Work out the finished part from the listing and answer in its coordinate system (mm). Round coordinates to 2 decimals unless told otherwise and drop trailing zeros. Loops run counter-clockwise (first coordinate to the right, second up) from the corner with the lowest first, then second, coordinate; pieces in that order, holes last. Notation, with made-up numbers: (32, -11.75) -> (50, -11.75) arc R21 ccw to (50, 0.25) -> close; hole circle Ø4 at (-19, 46). An arc over 180 degrees is marked (long way). Use one line per item in the form item = value.
Autodesk Inventor part; units mm, degrees
ref_plane "YZ Plane" through (0, 0, 0) normal (1, 0, 0) x (0, 1, 0)
ref_plane "XZ Plane" through (0, 0, 0) normal (0, 1, 0) x (-1, 0, 0)
ref_plane "XY Plane" through (0, 0, 0) normal (0, 0, 1) x (1, 0, 0)
sketch "Sketch1" plane through (0, 0, 0) normal (0, 1, 0) x (-1, 0, 0)
  line L0 (0, 0) -> (558.8, 0)
  line L1 (558.8, 0) -> (558.8, 79.375)
  line L2 (558.8, 79.375) -> (0, 79.375)
  line L3 (0, 79.375) -> (0, 0)
  dimension "d0" = 79.375
  dimension "d1" = 558.8
extrude "Extrusion1" add sketch "Sketch1" along normal blind 3.175
sketch "Sketch3" plane through (-558.8, 0, 0) normal (-1, 0, 0) x (0, 0, 1)
  line L0 (0, 0) -> (79.375, 0)
  line L1 (79.375, 0) -> (79.375, 3.175)
  line L2 (0, 3.175) -> (79.375, 3.175)
  line L3 (0, 0) -> (0, 3.175)
  line L4 (73.025, 3.175) -> (73.025, 0)
  line L5 (60.325, 0) -> (60.325, 3.175)
  line L6 (19.05, 0) -> (19.05, 3.175)
  line L7 (6.35, 0) -> (6.35, 3.175)
  dimension "d4" = 12.7
  dimension "d5" = 6.35
  dimension "d6" = 12.7
  dimension "d7" = 6.35
extrude "Extrusion2" cut sketch "Sketch3" against normal blind 3.175 contours L7 L2 L6 L0 | L5 L2 L4 L0
sketch "Sketch4" plane through (0, 0, 79.375) normal (1, 0, 0) x (0, 0, -1)
  line L0 (19.05, 3.175) -> (6.35, 3.175)
  line L1 (19.05, 0) -> (19.05, 3.175)
  line L2 (6.35, 0) -> (19.05, 0)
  line L3 (6.35, 3.175) -> (6.35, 0)
  line L4 (60.325, 3.175) -> (60.325, 0)
  line L5 (73.025, 3.175) -> (60.325, 3.175)
  line L6 (73.025, 0) -> (73.025, 3.175)
  line L7 (60.325, 0) -> (73.025, 0)
extrude "Extrusion3" cut sketch "Sketch4" against normal blind 6.35
sketch "Sketch5" plane through (0, 0, 0) normal (0, -1, 0) x (1, 0, 0)
  line L0 (-558.8, 79.375) -> (0, 79.375)
  line L1 (-558.8, 19.05) -> (-558.8, 60.325)
  line L2 (0, 0) -> (-558.8, 0)
  line L3 (-542.925, 73.025) -> (-542.925, 6.35)
  line L4 (-542.925, 6.35) -> (-530.225, 6.35)
  line L5 (-542.925, 73.025) -> (-530.225, 73.025)
  line L6 (-530.225, 73.025) -> (-530.225, 6.35)
  line L7 (-517.525, 73.025) -> (-517.525, 6.35)
  line L8 (-517.525, 6.35) -> (-504.825, 6.35)
  line L9 (-517.525, 73.025) -> (-504.825, 73.025)
  line L10 (-504.825, 73.025) -> (-504.825, 6.35)
  line L11 (-492.125, 73.025) -> (-492.125, 6.35)
  line L12 (-492.125, 6.35) -> (-479.425, 6.35)
  line L13 (-492.125, 73.025) -> (-479.425, 73.025)
  line L14 (-479.425, 73.025) -> (-479.425, 6.35)
  line L15 (-466.725, 73.025) -> (-466.725, 6.35)
  line L16 (-466.725, 6.35) -> (-454.025, 6.35)
  line L17 (-466.725, 73.025) -> (-454.025, 73.025)
  line L18 (-454.025, 73.025) -> (-454.025, 6.35)
  line L19 (-441.325, 73.025) -> (-441.325, 6.35)
  line L20 (-441.325, 6.35) -> (-428.625, 6.35)
  line L21 (-441.325, 73.025) -> (-428.625, 73.025)
  line L22 (-428.625, 73.025) -> (-428.625, 6.35)
  line L23 (-415.925, 73.025) -> (-415.925, 6.35)
  line L24 (-415.925, 6.35) -> (-403.225, 6.35)
  line L25 (-415.925, 73.025) -> (-403.225, 73.025)
  line L26 (-403.225, 73.025) -> (-403.225, 6.35)
  line L27 (-390.525, 73.025) -> (-390.525, 6.35)
  line L28 (-390.525, 6.35) -> (-377.825, 6.35)
  line L29 (-390.525, 73.025) -> (-377.825, 73.025)
  line L30 (-377.825, 73.025) -> (-377.825, 6.35)
  line L31 (-365.125, 73.025) -> (-365.125, 6.35)
  line L32 (-365.125, 6.35) -> (-352.425, 6.35)
  line L33 (-365.125, 73.025) -> (-352.425, 73.025)
  line L34 (-352.425, 73.025) -> (-352.425, 6.35)
  line L35 (-339.725, 73.025) -> (-339.725, 6.35)
  line L36 (-339.725, 6.35) -> (-327.025, 6.35)
  line L37 (-339.725, 73.025) -> (-327.025, 73.025)
  line L38 (-327.025, 73.025) -> (-327.025, 6.35)
  line L39 (-314.325, 73.025) -> (-314.325, 6.35)
  line L40 (-314.325, 6.35) -> (-301.625, 6.35)
  line L41 (-314.325, 73.025) -> (-301.625, 73.025)
  line L42 (-301.625, 73.025) -> (-301.625, 6.35)
  line L43 (-288.925, 73.025) -> (-288.925, 6.35)
  line L44 (-288.925, 6.35) -> (-276.225, 6.35)
  line L45 (-288.925, 73.025) -> (-276.225, 73.025)
  line L46 (-276.225, 73.025) -> (-276.225, 6.35)
  line L47 (-263.525, 73.025) -> (-263.525, 6.35)
  line L48 (-263.525, 6.35) -> (-250.825, 6.35)
  line L49 (-263.525, 73.025) -> (-250.825, 73.025)
  line L50 (-250.825, 73.025) -> (-250.825, 6.35)
  line L51 (-238.125, 73.025) -> (-238.125, 6.35)
  line L52 (-238.125, 6.35) -> (-225.425, 6.35)
  line L53 (-238.125, 73.025) -> (-225.425, 73.025)
  line L54 (-225.425, 73.025) -> (-225.425, 6.35)
  line L55 (-212.725, 73.025) -> (-212.725, 6.35)
  line L56 (-212.725, 6.35) -> (-200.025, 6.35)
  line L57 (-212.725, 73.025) -> (-200.025, 73.025)
  line L58 (-200.025, 73.025) -> (-200.025, 6.35)
  line L59 (-187.325, 73.025) -> (-187.325, 6.35)
  line L60 (-187.325, 6.35) -> (-174.625, 6.35)
  line L61 (-187.325, 73.025) -> (-174.625, 73.025)
  line L62 (-174.625, 73.025) -> (-174.625, 6.35)
  line L63 (-161.925, 73.025) -> (-161.925, 6.35)
  line L64 (-161.925, 6.35) -> (-149.225, 6.35)
  line L65 (-161.925, 73.025) -> (-149.225, 73.025)
  line L66 (-149.225, 73.025) -> (-149.225, 6.35)
  line L67 (-136.525, 73.025) -> (-136.525, 6.35)
  line L68 (-136.525, 6.35) -> (-123.825, 6.35)
  line L69 (-136.525, 73.025) -> (-123.825, 73.025)
  line L70 (-123.825, 73.025) -> (-123.825, 6.35)
  line L71 (-111.125, 73.025) -> (-111.125, 6.35)
  line L72 (-111.125, 6.35) -> (-98.425, 6.35)
  line L73 (-111.125, 73.025) -> (-98.425, 73.025)
  line L74 (-98.425, 73.025) -> (-98.425, 6.35)
  line L75 (-85.725, 73.025) -> (-85.725, 6.35)
  line L76 (-85.725, 6.35) -> (-73.025, 6.35)
  line L77 (-85.725, 73.025) -> (-73.025, 73.025)
  line L78 (-73.025, 73.025) -> (-73.025, 6.35)
  line L79 (-60.325, 73.025) -> (-60.325, 6.35)
  line L80 (-60.325, 6.35) -> (-47.625, 6.35)
  line L81 (-60.325, 73.025) -> (-47.625, 73.025)
  line L82 (-47.625, 73.025) -> (-47.625, 6.35)
  line L83 (-34.925, 73.025) -> (-34.925, 6.35)
  line L84 (-34.925, 6.35) -> (-22.225, 6.35)
  line L85 (-34.925, 73.025) -> (-22.225, 73.025)
  line L86 (-22.225, 73.025) -> (-22.225, 6.35)
  dimension "d12" = 12.7
  dimension "d14" = 15.875
  dimension "d15" = 6.35
  dimension "d16" = 6.35
  dimension "d19" = 25.4
extrude "Extrusion4" cut sketch "Sketch5" against normal blind 25.4 contours L5 L6 L4 L3 | L9 L10 L8 L7 | L13 L14 L12 L11 | L17 L18 L16 L15 | L21 L22 L20 L19 | L25 L26 L24 L23 | L29 L30 L28 L27 | L33 L34 L32 L31 | L37 L38 L36 L35 | L45 L46 L44 L43 | L49 L50 L48 L47 | L53 L54 L52 L51 | L57 L58 L56 L55 | L61 L62 L60 L59 | L65 L66 L64 L63 | L69 L70 L68 L67 | L73 L74 L72 L71 | L77 L78 L76 L75 | L81 L82 L80 L79 | L85 L86 L84 L83
sketch "Sketch6" plane through (0, 0, 0) normal (0, -1, 0) x (1, 0, 0)
  line L0 (0, 60.325) -> (-6.35, 60.325)
  line L1 (-6.35, 60.325) -> (-6.35, 73.025)
  line L2 (-6.35, 73.025) -> (0, 73.025)
  line L3 (0, 79.375) -> (0, 73.025)
  line L4 (-558.8, 79.375) -> (0, 79.375)
  line L5 (0, 60.325) -> (0, 19.05)
  line L6 (0, 60.325) -> (0, 73.025)
  line L7 (-25.4, 79.375) -> (0, 49.1045)
  dimension "d26" = 50
  dimension "d27" = 25.4
extrude "Extrusion5" cut sketch "Sketch6" against normal blind 25.4 contours L5 L7 L4 L3 L2 L1 L0
properties part number "Wing" material "Polycarbonate, Clear"
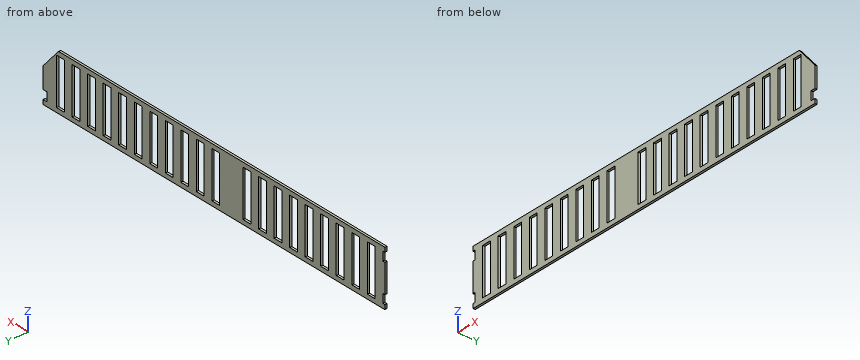
(1) Given P1, Ø1, axis at y = 2, z = 10.5, coming from the +X side, flat-ended and moving along its own axis, determine where the tip first touches the part or whether it passes through.
Completed:
P1 = -6.35
(2) Find section B-B, the plane z = 39. State how many separate pieces and enclosed holes the cut face has, then the cut area to 3 significant figures.
Completed:
separate_pieces = 21
enclosed_holes = 0
area = 968 mm2
(3) Consider L1, parallel to Z at x = -83, y = 2.6 (3 decimals); L2, parallel to X at y = 2.3, z = 73.5; L3, parallel to X at y = 2.6, z = 76. Determine where each line is inside the solid, lowest interval first.
Completed:
L1 = 0 to 6.35, 73.025 to 79.375
L2 = -558.8 to -20.47
L3 = -558.8 to -22.57
(4) Find section A-A, the plane x = -359.5. Write down the section's boundary in (y, z) (3 decimals), then the cut area to 3 significant figures.
Completed:
outline = (0, 0) -> (3.175, 0) -> (3.175, 6.35) -> (0, 6.35) -> close; (0, 73.025) -> (3.175, 73.025) -> (3.175, 79.375) -> (0, 79.375) -> close
area = 40.3 mm2
